```python
from build123d import *

# Parameters (mm, degrees)
SKETCH1_W           = 160
SKETCH1_H           = 160
BOSS_EXTRUDE1_DEPTH = 1.25
SKETCH3_W           = 2.5
SKETCH3_H           = 10
SKETCH3_W_2         = 10
SKETCH3_H_2         = 2.5
CUT_EXTRUDE2_DEPTH  = 114.164702978
SKETCH2_R           = 1.5
CUT_EXTRUDE1_DEPTH  = 114.164702978


with BuildPart() as part:
    # Sketch1 → Boss-Extrude1 (new, symmetric)
    with BuildSketch(Plane(origin=(0, 0, 0), x_dir=(1, 0, 0), z_dir=(0, 1, 0))):
        Rectangle(SKETCH1_W, SKETCH1_H)
    extrude(amount=BOSS_EXTRUDE1_DEPTH, both=True)

    # Sketch3 → Cut-Extrude2 (cut, through all)
    with BuildSketch(Plane(origin=(0, 1.25, 0), x_dir=(1, 0, 0), z_dir=(0, 1, 0))):
        with Locations((-78.75, 60)):
            Rectangle(SKETCH3_W, SKETCH3_H)
        with Locations((-78.75, 40)):
            Rectangle(SKETCH3_W, SKETCH3_H)
        with Locations((-78.75, 20)):
            Rectangle(SKETCH3_W, SKETCH3_H)
        with Locations((-78.75, 0)):
            Rectangle(SKETCH3_W, SKETCH3_H)
        with Locations((-78.75, -20)):
            Rectangle(SKETCH3_W, SKETCH3_H)
        with Locations((-78.75, -40)):
            Rectangle(SKETCH3_W, SKETCH3_H)
        with Locations((-78.75, -60)):
            Rectangle(SKETCH3_W, SKETCH3_H)
        with Locations((-60, -78.75)):
            Rectangle(SKETCH3_W_2, SKETCH3_H_2)
        with Locations((-40, -78.75)):
            Rectangle(SKETCH3_W_2, SKETCH3_H_2)
        with Locations((-20, -78.75)):
            Rectangle(SKETCH3_W_2, SKETCH3_H_2)
        with Locations((0, -78.75)):
            Rectangle(SKETCH3_W_2, SKETCH3_H_2)
        with Locations((20, -78.75)):
            Rectangle(SKETCH3_W_2, SKETCH3_H_2)
        with Locations((40, -78.75)):
            Rectangle(SKETCH3_W_2, SKETCH3_H_2)
        with Locations((60, -78.75)):
            Rectangle(SKETCH3_W_2, SKETCH3_H_2)
        with Locations((78.75, -60)):
            Rectangle(SKETCH3_W, SKETCH3_H)
        with Locations((78.75, 40)):
            Rectangle(SKETCH3_W, SKETCH3_H)
        with Locations((78.75, 20)):
            Rectangle(SKETCH3_W, SKETCH3_H)
        with Locations((78.75, 0)):
            Rectangle(SKETCH3_W, SKETCH3_H)
        with Locations((78.75, -20)):
            Rectangle(SKETCH3_W, SKETCH3_H)
        with Locations((78.75, -40)):
            Rectangle(SKETCH3_W, SKETCH3_H)
        with Locations((60, 78.75)):
            Rectangle(SKETCH3_W_2, SKETCH3_H_2)
        with Locations((40, 78.75)):
            Rectangle(SKETCH3_W_2, SKETCH3_H_2)
        with Locations((20, 78.75)):
            Rectangle(SKETCH3_W_2, SKETCH3_H_2)
        with Locations((0, 78.75)):
            Rectangle(SKETCH3_W_2, SKETCH3_H_2)
        with Locations((-20, 78.75)):
            Rectangle(SKETCH3_W_2, SKETCH3_H_2)
        with Locations((-40, 78.75)):
            Rectangle(SKETCH3_W_2, SKETCH3_H_2)
        with Locations((-60, 78.75)):
            Rectangle(SKETCH3_W_2, SKETCH3_H_2)
        with Locations((78.75, 60)):
            Rectangle(SKETCH3_W, SKETCH3_H)
    extrude(amount=-CUT_EXTRUDE2_DEPTH, mode=Mode.SUBTRACT)

    # Sketch2 → Cut-Extrude1 (cut, through all)
    with BuildSketch(Plane(origin=(0, 1.25, 0), x_dir=(1, 0, 0), z_dir=(0, 1, 0))):
        with Locations(Location((24.35481, 66.99998, 0), (0, 0, 270))):
            Circle(SKETCH2_R)
        with Locations(Location((-70.50001, 66.99998, 0), (0, 0, 270))):
            Circle(SKETCH2_R)
        with Locations(Location((70.38235, -15.19905, 0), (0, 0, 270))):
            Circle(SKETCH2_R)
        with Locations(Location((-31.25208, 5.67683, 0), (0, 0, 270))):
            Circle(SKETCH2_R)
        with Locations(Location((3.45737, 5.67683, 0), (0, 0, 270))):
            Circle(SKETCH2_R)
        with Locations(Location((3.45737, -36.07493, 0), (0, 0, 270))):
            Circle(SKETCH2_R)
        with Locations(Location((-70.50001, -70.67262, 0), (0, 0, 270))):
            Circle(SKETCH2_R)
        with Locations(Location((-31.25208, -36.07493, 0), (0, 0, 270))):
            Circle(SKETCH2_R)
        with Locations(Location((70.38235, -70.67262, 0), (0, 0, 270))):
            Circle(SKETCH2_R)
    extrude(amount=-CUT_EXTRUDE1_DEPTH, mode=Mode.SUBTRACT)


solid = part.part
```
Model file for the job. Use its own axes, mm. Coordinates: 2 decimals unless noted, no trailing zeros. Write each loop counter-clockwise with the first axis right and the second up, starting at its lowest first coordinate (ties: lowest second). Pieces come first, ordered by that corner, then holes. Notation, with made-up numbers: (80.25, -17.5) - (126.25, -17.5) arc R28 cw to (126.25, 18.5) - close; hole circle Ø3 at (24, 79). An arc over 180 degrees is marked (long way). Use a Markdown table: item, result. Add a question column.
Item 1: Band-saw the part on A-A, the plane x = 59.5. Write the cut outline in (y, z), and give its area (4 significant figures).
Item 2: Band-saw the part on B-B, the plane z = -60.5. Write the cut outline in (x, y).
Item 3: Drill centre lines: line 1 along Z through (x, y) = (70, -0.35); line 2 along X through (y, z) = (0.4, 0); line 3 along X through (y, z) = (-1, -67.5). Where is each one in solid material? Low to high.
Item 4: Drop flat-ended pins along their axis: pin 1 (1 mm diameter, centred on y = 1, z = -41, fed in from +X); pin 2 (1.2 mm diameter, centred on x = -18.5, y = -0.5, fed in from +Z). Give the stop position or say it passes through.
Item 5: Band-saw the part on C-C, the plane y = 0.7. Give the number of separate pieces and of enclosed holes in the cut face, and give its area (3 significant figures).
A:
| question | item | result |
|---|---|---|
| 1 | outline | (-1.25, -77.5) - (1.25, -77.5) - (1.25, 77.5) - (-1.25, 77.5) - close |
| 1 | area | 387.5 mm² |
| 2 | outline | (-77.5, -1.25) - (77.5, -1.25) - (77.5, 1.25) - (-77.5, 1.25) - close |
| 3 | line 1 | z = -80 to 13.75, 16.65 to 69.22, 72.12 to 80 |
| 3 | line 2 | x = -77.5 to 77.5 |
| 3 | line 3 | x = -80 to -71.91, -69.09 to 22.94, 25.77 to 80 |
| 4 | pin 1 | stops at x = 77.5 |
| 4 | pin 2 | stops at z = 77.5 |
| 5 | separate pieces | 1 |
| 5 | enclosed holes | 9 |
| 5 | area | 24,800 mm² |
